```python
from build123d import *

# Parameters (mm, degrees)
F0_W      = 137
F0_H      = 60
F0_W_2    = 127
F0_H_2    = 50
F1_DEPTH  = 25
F3_DEPTH  = 137.001
F4_DEPTH  = 10
F6_DEPTH  = 17.5
F7_W      = 137
F7_H      = 5
F8_DEPTH  = 7.5
F11_DEPTH = 137.001
F12_DEPTH = 5
F14_DEPTH = 137.001
F9_W      = 127
F9_H      = 15
F15_DEPTH = 57.001
F17_DEPTH = 137.001
F18_DEPTH = 5
F20_DEPTH = 5
F22_DEPTH = 5


with BuildPart() as f1:
    # F0 (on Top) → F1 (new body)
    with BuildSketch(Plane.XY):
        Rectangle(F0_W, F0_H)
        Rectangle(F0_W_2, F0_H_2, mode=Mode.SUBTRACT)
    extrude(amount=F1_DEPTH)

    # F2 (on face) → F3 (cut, through all)
    with BuildSketch(Plane(origin=(-68.5, 0, 0), x_dir=(0, -1, 0), z_dir=(-1, 0, 0))):
        Polygon((30, 25), (-25, 25), (30, 5), align=None)
    extrude(amount=-F3_DEPTH, mode=Mode.SUBTRACT)

    # F4 (add): a face of the model
    f4_faces = [f1.faces().sort_by_distance(p)[0] for p in [
        (0, 30, 12.5),
    ]]
    extrude(f4_faces, amount=F4_DEPTH)

    # F5 (on face) → F6 (join)
    with BuildSketch(Plane.XY.offset(25)):
        Polygon((68.5, 32.5), (-68.5, 32.5), (-68.5, 25), (-63.5, 25), (63.5, 25), (68.5, 25), align=None)
    extrude(amount=F6_DEPTH)

    # F7 (on face) → F8 (join, through all)
    with BuildSketch(Plane(origin=(0, 32.5, 0), x_dir=(-1, 0, 0), z_dir=(0, 1, 0))):
        with Locations((0, 40)):
            Rectangle(F7_W, F7_H)
    extrude(amount=F8_DEPTH)

    # F10 (on face) → F11 (cut, through all)
    with BuildSketch(Plane.YZ.offset(68.5)):
        Polygon((-30, 0), (-17, 0), (-17, 9.7272727273), (-30, 5), align=None)
    extrude(amount=-F11_DEPTH, mode=Mode.SUBTRACT)

    # F12 (cut): a face of the model
    f12_faces = [f1.faces().sort_by_distance(p)[0] for p in [
        (0, 25, 21.6425527142),
    ]]
    extrude(f12_faces, amount=-F12_DEPTH, mode=Mode.SUBTRACT)

    # F13 (on face) → F14 (cut, through all)
    with BuildSketch(Plane(origin=(-68.5, 0, 0), x_dir=(0, -1, 0), z_dir=(-1, 0, 0))):
        Polygon((-25, 25), (17, 5), (17, 9.7272727273), align=None)
    extrude(amount=-F14_DEPTH, mode=Mode.SUBTRACT)

    # F9 (on face) → F15 (cut, through all)
    with BuildSketch(Plane(origin=(0, 40, 0), x_dir=(-1, 0, 0), z_dir=(0, 1, 0))):
        with Locations((0, 12.5)):
            Rectangle(F9_W, F9_H)
    extrude(amount=-F15_DEPTH, mode=Mode.SUBTRACT)

    # F16 (on face) → F17 (cut, through all)
    with BuildSketch(Plane(origin=(-68.5, 0, 0), x_dir=(0, -1, 0), z_dir=(-1, 0, 0))):
        Polygon((5.3702966504, 5), (-9.2771325107, 11.9749662672), (-26.1297033496, 20), (-35, 20), (-35, 5), align=None)
    extrude(amount=-F17_DEPTH, mode=Mode.SUBTRACT)

    # F18 (cut, through all): a face of the model
    f18_faces = [f1.faces().sort_by_distance(p)[0] for p in [
        (0, 30, 2.5),
    ]]
    extrude(f18_faces, amount=-F18_DEPTH, mode=Mode.SUBTRACT)

    # F19 (on face) → F20 (join)
    with BuildSketch(Plane(origin=(-68.5, 0, 0), x_dir=(0, -1, 0), z_dir=(-1, 0, 0))):
        Polygon((-35, 5), (-30, 5), (-35, 10), align=None)
    extrude(amount=-F20_DEPTH)

    # F21 (on face) → F22 (join)
    with BuildSketch(Plane.YZ.offset(68.5)):
        Polygon((35, 10), (30, 5), (35, 5), align=None)
    extrude(amount=-F22_DEPTH)


solid = f1.part
```
The listing builds one solid part. Answer for the finished solid, in the listing's coordinates (mm). A direction names the side the tool comes from. Give positions to 0.01 mm unless a question says otherwise; leave off trailing zeros. Order: outer loops, then holes, each group sorted by start corner. A loop starts at its lowest first (then second) coordinate and runs counter-clockwise, first axis right, second up. Notation, with made-up numbers: (39, 38) - (82, 38) arc R13 ccw to (82, 42) - close; hole circle Ø6 at (27, -17.75). An arc over 180 degrees is marked (long way). Use one line per item in the form item = value. Start each with the question number.
(1) A cutting plane is placed at C-C, the plane z = 7. Write down the section's boundary in (x, y).
(2) For faces 5 (the flat face through (65.965, 10.159, 12.395)), 6 (the flat face through (-63.5, 12, 4)), 7 (the flat face through (-1, 35, 2)), 8 (the flat face through (-1, 36, 25)), determine the directions among +Z, -Z, +X, -X, +Y, -Y from which every point of the face is accessible in a straight line to the end or side of a thin tool.
(3) Consider line 1 (Z direction, x = 38, y = 37.5); line 2 (X direction, y = -4.5, z = 8); line 3 (Y direction, x = 44, z = 39.5). Determine where each line is inside the solid, lowest interval first. Write a range as from..to.
(4) A cutting plane is placed at B-B, the plane y = 20. Write down the section's boundary in (x, z), then the cut area to 3 significant figures.
(5) The mould has two halves that part along Z. Classify faces 1 (the flat face through (1, 35, 42.5)), 2 (the flat face through (68.5, 18, 17)), 3 (the flat face through (66, 13, 5)), 4 (the flat face through (1, 32.5, 31)): released by +Z, released by -Z, zero draft, split by the parting line, or undercut.
(6) A cutting plane is placed at A-A, the plane x = -36.5. Write down the section's boundary in (y, z).
(7) Flat-ended cylindrical pins translate along their axes: pin 1 Ø4 at (x, y) = (-65.5, 5) entering from +Z; pin 2 Ø5.5 at (x, z) = (66, 17.5) entering from -Y (3 decimals); pin 3 Ø10 at (x, z) = (52, 21.5) entering from -Y. Find the tip coordinate at first contact, or state that the pin passes through.
(8) A cutting plane is placed at D-D, the plane z = 34. Write down the section's boundary in (x, y).
Ans:
q1.outline = (-68.5, -12.8) - (-63.5, -12.8) - (-63.5, -1.17) - (-68.5, -1.17) - close; (-68.5, 32) - (-63.5, 32) - (-63.5, 40) - (-68.5, 40) - close; (63.5, -12.8) - (68.5, -12.8) - (68.5, -1.17) - (63.5, -1.17) - close; (63.5, 32) - (68.5, 32) - (68.5, 40) - (63.5, 40) - close
q2.face_5 = +X, -X
q2.face_6 = -Y
q2.face_7 = -Z, -Y
q2.face_8 = +X, -X, +Y
q3.line_1 = 0..5, 20..25, 37.5..42.5
q3.line_2 = -68.5..-63.5, 63.5..68.5
q3.line_3 = 30..40
q4.outline = (-68.5, 0) - (-63.5, 0) - (-63.5, 5) - (-68.5, 5) - close; (-68.5, 17.08) - (-63.5, 17.08) - (-63.5, 22.62) - (-68.5, 22.62) - close; (63.5, 0) - (68.5, 0) - (68.5, 5) - (63.5, 5) - close; (63.5, 17.08) - (68.5, 17.08) - (68.5, 22.62) - (63.5, 22.62) - close
q4.area = 105 mm^2
q5.face_1 = released by +Z
q5.face_2 = zero draft
q5.face_3 = undercut
q5.face_4 = undercut
q6.outline = (30, 20) - (40, 20) - (40, 25) - (32.5, 25) - (32.5, 37.5) - (40, 37.5) - (40, 42.5) - (30, 42.5) - close; (35, 0) - (40, 0) - (40, 5) - (35, 5) - close
q7.pin_1 = 16.43
q7.pin_2 = 3.475
q7.pin_3 = 30
q8.outline = (-68.5, 30) - (68.5, 30) - (68.5, 32.5) - (-68.5, 32.5) - close
